For this review, take the finished solid that the model builds, in its own axes (mm). A direction names the side the tool comes from. Round coordinates to 2 decimals unless told otherwise and drop trailing zeros. Loops run counter-clockwise (first coordinate to the right, second up) from the corner with the lowest first, then second, coordinate; pieces in that order, holes last. Notation, with made-up numbers: (-34.75, -11) -> (-18.75, -11) arc R27 cw to (-18.75, 13) -> close; hole circle Ø7 at (-28.75, 38). An arc over 180 degrees is marked (long way). One line per question, with ' | ' between items. Start each with the question number.
1. Consider section B-B (x = 29.5). Write out the cut boundary in (y, z).
2. For pin 1 Ø1 at (x, z) = (5, 5.5) entering from -Y; pin 2 Ø4 at (x, z) = (31, 4) entering from -Y; pin 3 Ø0.9 at (x, z) = (25, 5.5) entering from +Y; pin 4 Ø2 at (x, z) = (9, 2.5) entering from -Y, all flat-tipped, find the tip position at first contact; note any pin that passes through.
3. For faces 1 (the face through (26.5, 22, 4.1)), 2 (the face through (14, 14, 8)), 3 (the face through (12.43, 23.1, 3.94)), 4 (the face through (2.5, 9, 4)), list the 3-axis set-ups (+Z, -Z, +X, -X, +Y, -Y) from which the entire face can be reached by the end or side of a thin tool; tool diameter is ignored.
4. Consider section C-C (y = 20). Write out the cut boundary in (x, z).
5. Consider section A-A (y = 8.5). Write out the cut boundary in (x, z).
6. Wall thickness on line 1 along X through (y, z) = (13.75, 7); line 2 along Y through (x, z) = (29.5, 2.75); line 3 along Y through (x, z) = (25.5, 5.5): over which ranges is each line inside the solid? List them lowest first.
7. Draft analysis for pull direction Y (two halves, no side actions). For faces 5 (the face through (13, 26, 4)), 6 (the face through (31.83, 0.37, 4.06)), 7 (the face through (14, 27, 4)), 8 (the face through (25, 4.5, 4)), state which applies: pulls with the +Y half, pulls with the -Y half, needs draft (parallel to the pull), parting line crosses it, or undercut.
```python
from build123d import *

# Parameters (mm, degrees)
PAD_DEPTH    = 8
PAD001_DEPTH = 8
FILLET_R     = 3
FILLET001_R  = 0.5
CHAMFER_SIZE = 2.99
FILLET002_R  = 5
POCKET_DEPTH = 8.001
FILLET003_R  = 2


with BuildPart() as part:
    # Sketch → Pad (new body)
    with BuildSketch(Plane.XY):
        with BuildLine():
            Line((0, 0), (0, 28))
            Line((0, 28), (13, 28))
            Line((13, 28), (15, 26))
            Line((15, 26), (35, 26))
            Line((35, 26), (35, 23))
            Line((35, 23), (15, 23))
            Line((15, 23), (15, 3))
            Line((15, 3), (35, 3))
            Line((35, 3), (35, 0))
            Line((9.679449, 0), (35, 0))
            ThreePointArc((9.679449, 0), (11.736582, 1.844557), (12.5, 4.5))
            Line((12.5, 14.5), (12.5, 4.5))
            ThreePointArc((12.5, 14.5), (7.5, 19.5), (2.5, 14.5))
            Line((2.5, 4.5), (2.5, 14.5))
            ThreePointArc((2.5, 4.5), (3.263418, 1.844557), (5.320551, 0))
            Line((0, 0), (5.320551, 0))
        make_face()
    extrude(amount=PAD_DEPTH)

    # Sketch001 (on Face18 of Pad) → Pad001 (join)
    with BuildSketch(Plane.XY.offset(8)):
        Polygon((23, 23), (27, 23), (27, 22.5), (26, 21.5), (23, 21.5), align=None)
        Polygon((23, 3), (27, 3), (27, 3.5), (26, 4.5), (23, 4.5), align=None)
    extrude(amount=-PAD001_DEPTH)

    # Fillet
    fillet_edges = [part.edges().sort_by_distance(p)[0] for p in [
        (0, 0, 4),
        (0, 28, 4),
    ]]
    fillet(fillet_edges, radius=FILLET_R)

    # Fillet001
    fillet001_edges = [part.edges().sort_by_distance(p)[0] for p in [
        (15, 26, 4),
        (13, 28, 4),
        (5.320551, 0, 4),
        (9.679449, 0, 4),
    ]]
    fillet(fillet001_edges, radius=FILLET001_R)

    # Chamfer
    chamfer_edges = [part.edges().sort_by_distance(p)[0] for p in [
        (35, 26, 4),
        (35, 0, 4),
    ]]
    chamfer(chamfer_edges, length=CHAMFER_SIZE)

    # Fillet002
    fillet002_edges = [part.edges().sort_by_distance(p)[0] for p in [
        (32.01, 26, 4),
        (32.01, 0, 4),
    ]]
    fillet(fillet002_edges, radius=FILLET002_R)

    # Sketch002 (on Face32 of Fillet002) → Pocket (cut, through all)
    with BuildSketch(Plane.XY.offset(8)):
        with BuildLine():
            Line((9.5, 28), (11, 26.5))
            Line((11, 26.5), (3.5, 26.5))
            ThreePointArc((3.5, 26.5), (1.5, 24.5), (3.5, 22.5))
            Line((3.5, 22.5), (13, 22.5))
            Line((13, 22.5), (13, 28))
            Line((9.5, 28), (13, 28))
        make_face()
    extrude(amount=-POCKET_DEPTH, mode=Mode.SUBTRACT)

    # Fillet003
    fillet003_edges = [part.edges().sort_by_distance(p)[0] for p in [
        (13, 22.5, 4),
    ]]
    fillet(fillet003_edges, radius=FILLET003_R)


solid = part.part
```
Answer block:
1) outline: (0, 0) -> (3, 0) -> (3, 8) -> (0, 8) -> close; (23, 0) -> (26, 0) -> (26, 8) -> (23, 8) -> close
2) pin 1: stops at y = 18.5 | pin 2: stops at y = 0 | pin 3: stops at y = 26 | pin 4: stops at y = 18.83
3) face 1: +Z, -Z, +X | face 2: +Z, +X, -X, +Y, -Y | face 3: +Z, -Z, +Y | face 4: +Z, -Z
4) outline: (0, 0) -> (15, 0) -> (15, 8) -> (0, 8) -> close
5) outline: (0, 0) -> (2.5, 0) -> (2.5, 8) -> (0, 8) -> close; (12.5, 0) -> (15, 0) -> (15, 8) -> (12.5, 8) -> close
6) line 1: x = 0 to 2.5, 12.5 to 15 | line 2: y = 0 to 3, 23 to 26 | line 3: y = 0 to 4.5, 21.5 to 26
7) face 5: needs draft | face 6: pulls with the -Y half | face 7: pulls with the +Y half | face 8: undercut
